Geometry check sheet. Reference: the model listing, model coordinates, mm. Give positions to 0.01 mm unless a question says otherwise; leave off trailing zeros. Loops run counter-clockwise (first coordinate to the right, second up) from the corner with the lowest first, then second, coordinate; pieces in that order, holes last.
1. Go/stop test with a flat-tipped pin: pin 1 Ø0.9 at (x, z) = (18.5, 6) entering from -Y. Record where the tip stops, or that it passes through.
2. Release check for a two-part mould opening along X. For faces 1 (the cylindrical face through (12.21, 45.73, 6.26)), 2 (the flat face through (-24, -39, 6)), 3 (the flat face through (1, 62, 6)) record: +X half, -X half, draft (parallel to the pull), parting line (faces both ways), or undercut.
3. Material ranges on L1, parallel to Y at x = -12.5, z = 10; L2, parallel to X at y = -133.5, z = 6.35; L3, parallel to Z at x = -16, y = -123, recorded low to high.
4. Cross-section at A-A, the plane x = -12.5. Record the cut outline in (y, z).
from build123d import *

# Parameters (mm, degrees)
CROQUIS1_W              = 50.8
CROQUIS1_H              = 200
CROQUIS1_R              = 2.25
SALIENTE_EXTRUIR1_DEPTH = 12.7
CROQUIS2_R              = 1.5
CORTAR_EXTRUIR1_DEPTH   = 20


with BuildPart() as part:
    # Croquis1 → Saliente-Extruir1 (new body)
    with BuildSketch(Plane.XY):
        with Locations((1.4, -38)):
            Rectangle(CROQUIS1_W, CROQUIS1_H)
        with Locations((-12.5, 43.5)):
            Circle(CROQUIS1_R, mode=Mode.SUBTRACT)
        with Locations((12.5, 43.5)):
            Circle(CROQUIS1_R, mode=Mode.SUBTRACT)
        with Locations((12.5, 18.5)):
            Circle(CROQUIS1_R, mode=Mode.SUBTRACT)
        with Locations((-12.5, 18.5)):
            Circle(CROQUIS1_R, mode=Mode.SUBTRACT)
    extrude(amount=SALIENTE_EXTRUIR1_DEPTH)

    # Croquis2 → Cortar-Extruir1 (cut)
    with BuildSketch(Plane.XZ.offset(138)):
        with Locations(Location((-16.1, 6.35, 0), (0, 0, 270))):
            Circle(CROQUIS2_R)
        with Locations(Location((18.9, 6.35, 0), (0, 0, 270))):
            Circle(CROQUIS2_R)
    extrude(amount=-CORTAR_EXTRUIR1_DEPTH, mode=Mode.SUBTRACT)


solid = part.part
Result:
1. pin 1: stops at y = -118
2. face 1: undercut
2. face 2: -X half
2. face 3: draft
3. L1: y = -138 to 16.25, 20.75 to 41.25, 45.75 to 62
3. L2: x = -24 to -17.6, -14.6 to 17.4, 20.4 to 26.8
3. L3: z = 0 to 4.85, 7.85 to 12.7
4. outline: (-138, 0) - (16.25, 0) - (16.25, 12.7) - (-138, 12.7) - close; (20.75, 0) - (41.25, 0) - (41.25, 12.7) - (20.75, 12.7) - close; (45.75, 0) - (62, 0) - (62, 12.7) - (45.75, 12.7) - close
